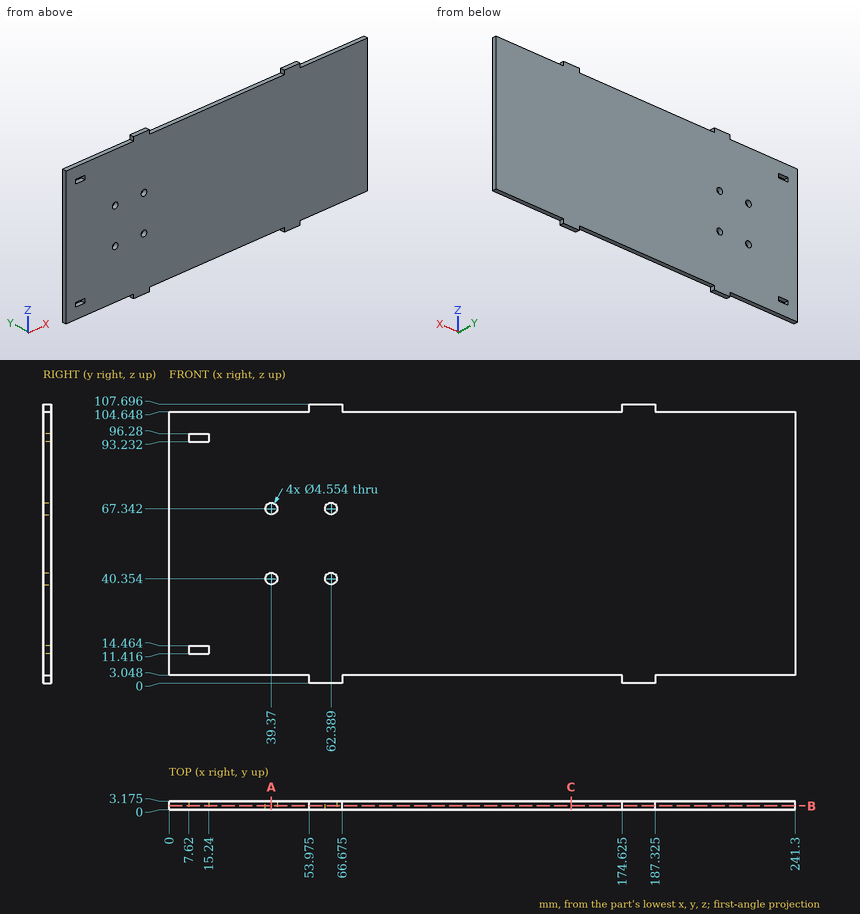
Check sheet for the drawn part. Datum: minimum x, y, z corner. Units: mm. Round coordinates to 2 decimals unless told otherwise and drop trailing zeros. Order: outer loops, then holes, each group sorted by start corner. A loop starts at its lowest first (then second) coordinate and runs counter-clockwise, first axis right, second up. Notation, with made-up numbers: (-15, -19) -> (40, -19) arc R10 ccw to (40, -11) -> close; hole circle Ø7 at (-6, 82.25). An arc over 180 degrees is marked (long way). Return JSON: item names as keys, results as strings. Group by question number.
Q1. Section check A-A, the plane x = 39.37. Record the boundary of the cut face in (y, z) (1 decimal), plus the area to 3 significant figures.
Q2. Gauge pin test, flat ends, axial feed: pin 1 (1.5 mm diameter, centred on y = 2, z = 1.5, fed in from -X) (3 decimals); pin 2 (1.6 mm diameter, centred on x = 211, y = 2.5, fed in from +Z); pin 3 (0.9 mm diameter, centred on y = 1, z = 106.5, fed in from +X) (3 decimals). Record the tip position at first contact, or that the pin passes through.
Q3. Section check B-B, the plane y = 1.45. Count the separate pieces of the cut face and the enclosed holes in it, plus the area to 3 significant figures.
Q4. Material ranges on probe 1 along Z at (x, y) = (39.37, 1.7) (1 decimal); probe 2 along Z at (x, y) = (77, 1.8); probe 3 along X at (y, z) = (1.35, 68.5), recorded low to high. Write a range as from..to.
Q5. Section check C-C, the plane x = 155. Record the boundary of the cut face in (y, z) (1 decimal).
Numbers:
{
 "1": {"outline": "(0, 3) -> (3.2, 3) -> (3.2, 38.1) -> (0, 38.1) -> close; (0, 42.6) -> (3.2, 42.6) -> (3.2, 65.1) -> (0, 65.1) -> close; (0, 69.6) -> (3.2, 69.6) -> (3.2, 104.6) -> (0, 104.6) -> close", "area": "294 mm^2"},
 "2": {"pin 1": "x = 53.975", "pin 2": "z = 104.65", "pin 3": "x = 187.325"},
 "3": {"separate pieces": "1", "enclosed holes": "6", "area": "24,600 mm^2"},
 "4": {"probe 1": "3..38.1, 42.6..65.1, 69.6..104.6", "probe 2": "3.05..104.65", "probe 3": "0..37.41, 41.33..60.43, 64.35..241.3"},
 "5": {"outline": "(0, 3) -> (3.2, 3) -> (3.2, 104.6) -> (0, 104.6) -> close"}
}
